Source: CAD feature listing. Evaluate the final solid. Frame: model axes, mm. A direction names the side the tool comes from. Round coordinates to 2 decimals unless told otherwise and drop trailing zeros. Write each loop counter-clockwise with the first axis right and the second up, starting at its lowest first coordinate (ties: lowest second). Pieces come first, ordered by that corner, then holes.
```python
from build123d import *

# Parameters (mm, degrees)
SKETCH1_R           = 1.5
BOSS_EXTRUDE1_DEPTH = 2


with BuildPart() as part:
    # Sketch1 → Boss-Extrude1 (new body)
    with BuildSketch(Plane(origin=(0, 0, 0), x_dir=(1, 0, 0), z_dir=(0, 1, 0))):
        Polygon((0, 0), (19.75, 0), (19.75, 26), (90.25, 26), (90.25, 0), (110, 0), (110, 25.5), (102, 33.5), (92.25, 33.5), (92.25, 35), (84.25, 43), (25.75, 43), (17.75, 35), (17.75, 33.5), (8, 33.5), (0, 25.5), align=None)
        with Locations(Location((10.25, 5, 0), (0, 0, 270))):
            Circle(SKETCH1_R, mode=Mode.SUBTRACT)
        with Locations(Location((34.75, 35, 0), (0, 0, 270))):
            Circle(SKETCH1_R, mode=Mode.SUBTRACT)
        with Locations(Location((75.25, 35, 0), (0, 0, 90))):
            Circle(SKETCH1_R, mode=Mode.SUBTRACT)
        with Locations(Location((99.75, 5, 0), (0, 0, 90))):
            Circle(SKETCH1_R, mode=Mode.SUBTRACT)
    extrude(amount=BOSS_EXTRUDE1_DEPTH)


solid = part.part
```
Q1. Section query C-C, the plane z = -5. Output: boundary loops of the cut face in (x, y).
Q2. Section query A-A, the plane y = 0.5. Output: boundary loops of the cut face in (x, z), and give its area (3 significant figures).
Q3. Pin query (flat end, axial travel): P1, Ø1, axis at x = 51, y = 1.5, coming from the +Z side; P2, Ø0.6, axis at x = 13, y = 1.5, coming from the -Z side; P3, Ø2.5, axis at x = 10.25, z = -5, coming from the +Y side. Return the tip coordinate at first contact, or that it passes through.
Q4. Section query B-B, the plane x = 99.75. Output: boundary loops of the cut face in (y, z), and give its area (3 significant figures).
Q5. Set-up query: faces 1 (the face through (97, 1, -33.5)), 2 (the face through (100, 1, 0)), 3 (the face through (19.75, 1, -13)). Return all of +Z, -Z, +X, -X, +Y, -Y with unobstructed straight access to the full face (end or side cutting, diameter ignored); none if empty.
Q6. Mould query, pull axis Z, two halves, no side actions, for faces 4 (the face through (13, 1, -33.5)), 5 (the face through (55, 1, -26)), 6 (the face through (9.34, 0.99, -6.19)). Classes: pulls with the +Z half, pulls with the -Z half, needs draft (parallel to the pull), parting line crosses it, or undercut.
Q7. Section query D-D, the plane z = -14.5. Output: boundary loops of the cut face in (x, y), and give its area (3 significant figures).
Q8. Line query: line 1 (X direction, y = 0.75, z = -5); line 2 (X direction, y = 1.5, z = -35); line 3 (X direction, y = 1.6, z = -23). Output: solid intervals per line, ascending.
Filled in:
1. outline: (0, 0) - (8.75, 0) - (8.75, 2) - (0, 2) - close; (11.75, 0) - (19.75, 0) - (19.75, 2) - (11.75, 2) - close; (90.25, 0) - (98.25, 0) - (98.25, 2) - (90.25, 2) - close; (101.25, 0) - (110, 0) - (110, 2) - (101.25, 2) - close
2. outline: (0, -25.5) - (8, -33.5) - (17.75, -33.5) - (17.75, -35) - (25.75, -43) - (84.25, -43) - (92.25, -35) - (92.25, -33.5) - (102, -33.5) - (110, -25.5) - (110, 0) - (90.25, 0) - (90.25, -26) - (19.75, -26) - (19.75, 0) - (0, 0) - close; hole circle Ø3 at (10.25, -5); hole circle Ø3 at (34.75, -35); hole circle Ø3 at (75.25, -35); hole circle Ø3 at (99.75, -5)
2. area: 2,400 mm2
3. P1: stops at z = -26
3. P2: stops at z = -33.5
3. P3: passes through
4. outline: (0, -33.5) - (2, -33.5) - (2, -6.5) - (0, -6.5) - close; (0, -3.5) - (2, -3.5) - (2, 0) - (0, 0) - close
4. area: 61.0 mm2
5. face 1: -Z, +X, +Y, -Y
5. face 2: +Z, +X, -X, +Y, -Y
5. face 3: +Z, +Y, -Y
6. face 4: pulls with the -Z half
6. face 5: pulls with the +Z half
6. face 6: undercut
7. outline: (0, 0) - (19.75, 0) - (19.75, 2) - (0, 2) - close; (90.25, 0) - (110, 0) - (110, 2) - (90.25, 2) - close
7. area: 79.0 mm2
8. line 1: x = 0 to 8.75, 11.75 to 19.75, 90.25 to 98.25, 101.25 to 110
8. line 2: x = 17.75 to 33.25, 36.25 to 73.75, 76.75 to 92.25
8. line 3: x = 0 to 19.75, 90.25 to 110
